from build123d import *

# Parameters (mm, degrees)
SKETCH1_W               = 50.8
SKETCH1_H               = 25.4
SKETCH1_W_2             = 44.45
SKETCH1_H_2             = 19.05
BOSS_EXTRUDE1_DEPTH     = 844.55
CUT_EXTRUDE1_DEPTH      = 847.457620026
CUT_EXTRUDE1_DEPTH_BACK = 847.457620026
SKETCH2_R               = 3.175
CUT_EXTRUDE2_DEPTH      = 847.457620026
CUT_EXTRUDE2_DEPTH_BACK = 847.457620026
SKETCH3_R               = 3.175
SKETCH4_R               = 3.175
CUT_EXTRUDE3_DEPTH      = 847.457620026
SKETCH5_R               = 3.175
CUT_EXTRUDE4_DEPTH      = 847.457620026


with BuildPart() as part:
    # Sketch1 → Boss-Extrude1 (new body)
    with BuildSketch(Plane.XY):
        with Locations((25.4, 12.7)):
            Rectangle(SKETCH1_W, SKETCH1_H)
        with Locations((25.4, 12.7)):
            Rectangle(SKETCH1_W_2, SKETCH1_H_2, mode=Mode.SUBTRACT)
    extrude(amount=BOSS_EXTRUDE1_DEPTH)

    # Sketch2 → Cut-Extrude1 (cut, two sides: drawn at the far end of the back side and taken through both)
    with BuildSketch(Plane(origin=(50.8, 0, 0), x_dir=(0, 0, -1), z_dir=(1, 0, 0)).offset(-CUT_EXTRUDE1_DEPTH_BACK)):
        with Locations((-76.2, 12.7)):
            Circle(SKETCH2_R)
        with Locations((-88.9, 12.7)):
            Circle(SKETCH2_R)
        with Locations((-101.6, 12.7)):
            Circle(SKETCH2_R)
    extrude(amount=CUT_EXTRUDE1_DEPTH + CUT_EXTRUDE1_DEPTH_BACK, mode=Mode.SUBTRACT)

    # Sketch3 → Cut-Extrude2 (cut, two sides: drawn at the far end of the back side and taken through both)
    with BuildSketch(Plane(origin=(0, 25.4, 0), x_dir=(1, 0, 0), z_dir=(0, 1, 0)).offset(-CUT_EXTRUDE2_DEPTH_BACK)):
        with Locations(Location((12.7, -19.05, 0), (0, 0, 270))):
            Circle(SKETCH3_R)
        with Locations(Location((25.4, -19.05, 0), (0, 0, 270))):
            Circle(SKETCH3_R)
        with Locations(Location((38.1, -19.05, 0), (0, 0, 270))):
            Circle(SKETCH3_R)
        with Locations(Location((25.4, -31.75, 0), (0, 0, 270))):
            Circle(SKETCH3_R)
        with Locations(Location((38.1, -31.75, 0), (0, 0, 270))):
            Circle(SKETCH3_R)
        with Locations(Location((25.4, -44.45, 0), (0, 0, 270))):
            Circle(SKETCH3_R)
        with Locations(Location((38.1, -44.45, 0), (0, 0, 270))):
            Circle(SKETCH3_R)
        with Locations(Location((12.7, -31.75, 0), (0, 0, 270))):
            Circle(SKETCH3_R)
        with Locations(Location((12.7, -44.45, 0), (0, 0, 270))):
            Circle(SKETCH3_R)
    extrude(amount=CUT_EXTRUDE2_DEPTH + CUT_EXTRUDE2_DEPTH_BACK, mode=Mode.SUBTRACT)

    # Sketch4 → Cut-Extrude3 (cut, through all)
    with BuildSketch(Plane(origin=(0, 25.4, 0), x_dir=(1, 0, 0), z_dir=(0, 1, 0))):
        with Locations(Location((12.7, -330.2, 0), (0, 0, 270))):
            Circle(SKETCH4_R)
        with Locations(Location((38.1, -330.2, 0), (0, 0, 270))):
            Circle(SKETCH4_R)
        with Locations(Location((12.7, -355.6, 0), (0, 0, 270))):
            Circle(SKETCH4_R)
        with Locations(Location((38.1, -355.6, 0), (0, 0, 270))):
            Circle(SKETCH4_R)
    extrude(amount=-CUT_EXTRUDE3_DEPTH, mode=Mode.SUBTRACT)

    # Sketch5 → Cut-Extrude4 (cut, through all)
    with BuildSketch(Plane(origin=(0, 25.4, 0), x_dir=(1, 0, 0), z_dir=(0, 1, 0))):
        with Locations(Location((12.7, -825.5, 0), (0, 0, 270))):
            Circle(SKETCH5_R)
        with Locations(Location((38.1, -825.5, 0), (0, 0, 270))):
            Circle(SKETCH5_R)
        with Locations(Location((38.1, -800.1, 0), (0, 0, 270))):
            Circle(SKETCH5_R)
        with Locations(Location((12.7, -800.1, 0), (0, 0, 270))):
            Circle(SKETCH5_R)
    extrude(amount=-CUT_EXTRUDE4_DEPTH, mode=Mode.SUBTRACT)


solid = part.part
Input: part model. Units: mm. Frame: model coordinates. A direction names the side the tool comes from. Give positions to 0.01 mm unless a question says otherwise; leave off trailing zeros. Order: outer loops, then holes, each group sorted by start corner. A loop starts at its lowest first (then second) coordinate and runs counter-clockwise, first axis right, second up. Notation, with made-up numbers: (-8.5, 22) - (27.5, 22) arc R14 cw to (27.5, 39) - close; hole circle Ø4 at (21.5, 73.5). An arc over 180 degrees is marked (long way). Write each question's results on one line, items separated by ' | '.
Item 1: Section A-A (z = 549.5). Return loops of the section in (x, y) (3 decimals).
A:
outline: (0, 0) - (50.8, 0) - (50.8, 25.4) - (0, 25.4) - close; hole (3.175, 3.175) - (47.625, 3.175) - (47.625, 22.225) - (3.175, 22.225) - close
Item 2: Access query for faces 4 (the flat face through (3.175, 13, 416)), 5 (the flat face through (25, 25.4, 416)). Directions: +Z, -Z, +X, -X, +Y, -Y. A direction counts if a zero-diameter tool reaches every point of the face in a straight line with its end or side. Return the directions, or none.
A:
face 4: +Z, -Z | face 5: +Z, -Z, +X, -X, +Y
Item 3: Material intervals for line 1 along X through (y, z) = (24.3, 330.2) (3 decimals); line 2 along X through (y, z) = (1.65, 44.45) (3 decimals); line 3 along X through (y, z) = (18.75, 481) (3 decimals), sorted ascending.
A:
line 1: x = 0 to 9.525, 15.875 to 34.925, 41.275 to 50.8 | line 2: x = 0 to 9.525, 15.875 to 22.225, 28.575 to 34.925, 41.275 to 50.8 | line 3: x = 0 to 3.175, 47.625 to 50.8
Item 4: Draft query along X for faces 1 (the flat face through (0, 13, 416)), 2 (the flat face through (25, 23, 0)), 3 (the flat face through (25, 22.225, 416)). Return one class per face: released by +X, released by -X, zero draft, split by the parting line, or undercut.
A:
face 1: released by -X | face 2: zero draft | face 3: undercut
